Can you work these out from the model? Positions are in its coordinate system, mm. Face numbers are marked on the shaded views. A direction names the side the tool comes from. Give positions to 0.01 mm unless a question says otherwise; leave off trailing zeros. Loops run counter-clockwise (first coordinate to the right, second up) from the corner with the lowest first, then second, coordinate; pieces in that order, holes last. Notation, with made-up numbers: (-36, -31.5) - (-19, -31.5) arc R30 ccw to (-19, -4.5) - close; hole circle Ø10 at (-22.75, -35). An arc over 180 degrees is marked (long way). Answer in a Markdown table with one row per item.
from build123d import *

# Parameters (mm, degrees)
PAD_DEPTH   = 15
FILLET_R    = 3
FILLET001_R = 2
FILLET002_R = 3
FILLET003_R = 1
FILLET004_R = 1
FILLET005_R = 4
FILLET006_R = 2
FILLET007_R = 1


with BuildPart() as part:
    # Sketch → Pad (new body)
    with BuildSketch(Plane.XZ):
        Polygon((38.909431, 83.441545), (38.909431, 0), (0, 0), (8.058298, 17.281077), (-8.54243, 20.208233), (-11.853996, 27.30991), (-8.543862, 27.30991), (-6.430771, 22.778371), (9.326153, 20), align=None)
        Polygon((35.909431, 69.90942), (4.709057, 3), (35.909431, 3), align=None, mode=Mode.SUBTRACT)
    extrude(amount=PAD_DEPTH)

    # Fillet
    fillet_edges = [part.edges().sort_by_distance(p)[0] for p in [
        (38.909431, -7.5, 0),
    ]]
    fillet(fillet_edges, radius=FILLET_R)

    # Fillet001
    fillet001_edges = [part.edges().sort_by_distance(p)[0] for p in [
        (0, -7.5, 0),
    ]]
    fillet(fillet001_edges, radius=FILLET001_R)

    # Fillet002
    fillet002_edges = [part.edges().sort_by_distance(p)[0] for p in [
        (38.909431, -7.5, 83.441545),
    ]]
    fillet(fillet002_edges, radius=FILLET002_R)

    # Fillet003
    fillet003_edges = [part.edges().sort_by_distance(p)[0] for p in [
        (35.909431, -7.5, 69.90942),
    ]]
    fillet(fillet003_edges, radius=FILLET003_R)

    # Fillet004
    fillet004_edges = [part.edges().sort_by_distance(p)[0] for p in [
        (4.709057, -7.5, 3),
    ]]
    fillet(fillet004_edges, radius=FILLET004_R)

    # Fillet005
    fillet005_edges = [part.edges().sort_by_distance(p)[0] for p in [
        (8.058298, -7.5, 17.281077),
    ]]
    fillet(fillet005_edges, radius=FILLET005_R)

    # Fillet006
    fillet006_edges = [part.edges().sort_by_distance(p)[0] for p in [
        (-6.430771, -7.5, 22.778371),
        (9.326153, -7.5, 20),
    ]]
    fillet(fillet006_edges, radius=FILLET006_R)

    # Fillet007
    fillet007_edges = [part.edges().sort_by_distance(p)[0] for p in [
        (-8.543862, -7.5, 27.30991),
        (-11.853996, -7.5, 27.30991),
        (-8.54243, -7.5, 20.208233),
    ]]
    fillet(fillet007_edges, radius=FILLET007_R)


solid = part.part
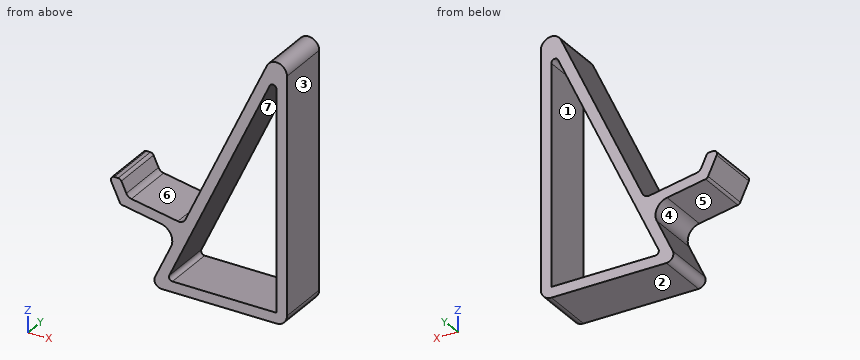
Q1. Imagine slicing it at B-B, the plane z = 47. Write out the boundary of the cut face in (x, y), and give its area (3 significant figures).
Checked values:
| item | result |
|---|---|
| outline | (21.92, -15) - (25.23, -15) - (25.23, 0) - (21.92, 0) - close; (35.91, -15) - (38.91, -15) - (38.91, 0) - (35.91, 0) - close |
| area | 94.7 mm² |
Q2. Imagine slicing it at C-C, the plane y = -2.25. Write out the boundary of the cut face in (x, z).
Checked values:
| item | result |
|---|---|
| outline | (-11.19, 25.89) - (-8.76, 20.68) arc R1 ccw to (-8.03, 20.12) - (2.92, 18.19) arc R4 cw to (5.86, 12.56) - (1.33, 2.85) arc R2 ccw to (3.14, 0) - (35.91, 0) arc R3 ccw to (38.91, 3) - (38.91, 69.91) arc R3 ccw to (33.19, 71.18) - (9.97, 21.39) arc R2 cw to (7.81, 20.27) - (-5.41, 22.6) arc R2 cw to (-6.87, 23.72) - (-8.27, 26.73) arc R1 ccw to (-9.18, 27.31) - (-10.28, 27.31) arc R1 ccw to start; hole (5.37, 4.42) arc R1 ccw to (6.28, 3) - (35.91, 3) - (35.91, 65.4) arc R1 ccw to (34, 65.82) - close |
Q3. On a 3-axis mill with a long thin cutter (end or side, diameter ignored), from which of +Z, -Z, +X, -X, +Y, -Y can I reach the whole of each face in a straight line? I mean the marked faces 5, 6 and 7. Say none if no direction works.
Checked values:
| item | result |
|---|---|
| face 5 | -X, +Y, -Y |
| face 6 | +Z, +Y, -Y |
| face 7 | +Y, -Y |
Q4. If we mould it in two halves opening along X, with no side actions, what happens to the marked faces 1, 2, 3 and 4? For each: released by +X, released by -X, zero draft, split by the parting line, or undercut.
Checked values:
| item | result |
|---|---|
| face 1 | undercut |
| face 2 | zero draft |
| face 3 | released by +X |
| face 4 | released by -X |
Q5. Imagine slicing it at A-A, the plane x = 35. Write out the boundary of the cut face in (y, z).
Checked values:
| item | result |
|---|---|
| outline | (-15, 0) - (0, 0) - (0, 3) - (-15, 3) - close; (-15, 66.39) - (0, 66.39) - (0, 72.77) - (-15, 72.77) - close |
Q6. Imagine slicing it at D-D, the plane x = -4. Write out the boundary of the cut face in (y, z), and give its area (3 significant figures).
Checked values:
| item | result |
|---|---|
| outline | (-15, 19.41) - (0, 19.41) - (0, 22.35) - (-15, 22.35) - close |
| area | 44.1 mm² |
Q7. If I drill on line 1 (X direction, y = -14, z = 25); line 2 (Z direction, x = 27, y = -5.5); line 3 (X direction, y = -13.25, z = 16.5), over which ranges is the centre line in solid material (lowest first)? Write a range as [from, to].
Checked values:
| item | result |
|---|---|
| line 1 | x = [-10.78, -7.47], [11.66, 14.97], [35.91, 38.91] |
| line 2 | z = [0, 3], [50.8, 57.9] |
| line 3 | x = [5.54, 11], [35.91, 38.91] |
Q8. For pin 1 (5 mm diameter, centred on y = -12.5, z = 8.5, fed in from -X); pin 2 (8 mm diameter, centred on y = -6, z = 13, fed in from -X); pin 3 (10 mm diameter, centred on x = -4.5, z = 28, fed in from +Y); pin 4 (0.6 mm diameter, centred on x = -9.5, y = -7.5, fed in from +Z), each with a flat end and sliding along its axis, tell me the tip position at first contact or that it passes through.
Checked values:
| item | result |
|---|---|
| pin 1 | stops at x = 2.8 |
| pin 2 | stops at x = 4.2 |
| pin 3 | stops at y = 0 |
| pin 4 | stops at z = 27.31 |
